Source: three-view drawing plus pictorial views. Frame: mm from the lowest corner of the part. Coordinates: 2 decimals unless noted, no trailing zeros. Write each loop counter-clockwise with the first axis right and the second up, starting at its lowest first coordinate (ties: lowest second). Pieces come first, ordered by that corner, then holes. Notation, with made-up numbers: (8, 69.25) -> (17, 69.25) arc R7 cw to (17, 80.25) -> close; hole circle Ø11 at (60.25, -6). An arc over 180 degrees is marked (long way). Write item = value, one per line.
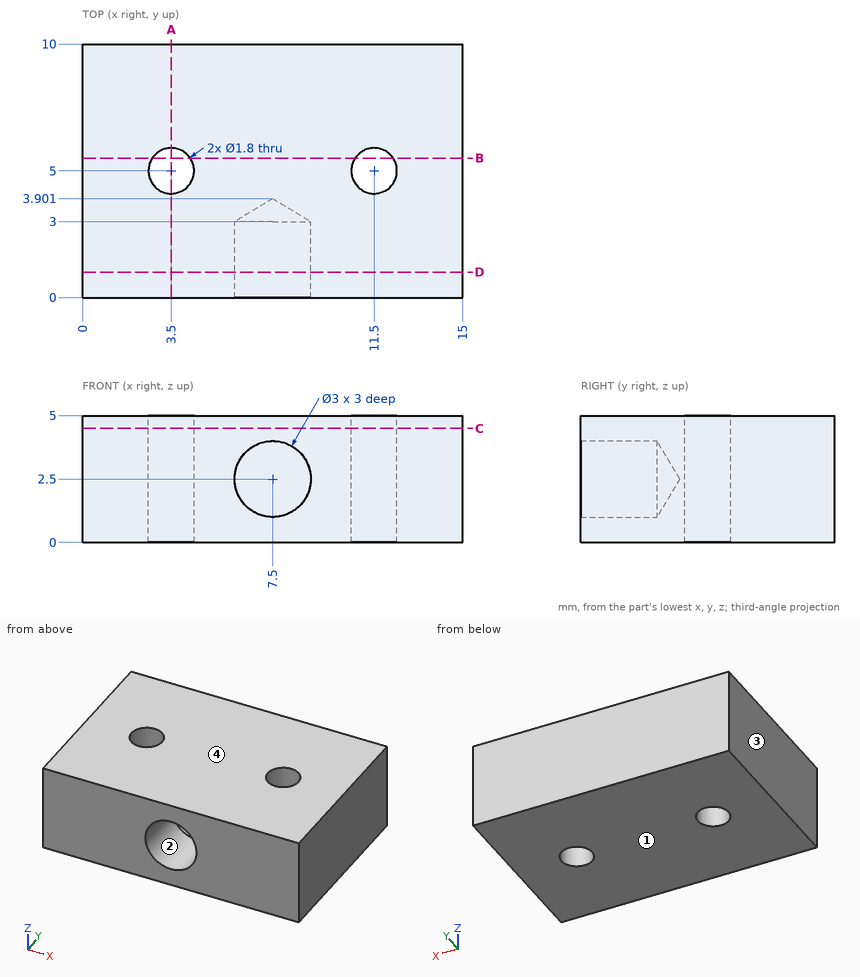
1) Cut plane A-A, the plane x = 3.5. Output: boundary loops of the cut face in (y, z), and give its area (3 significant figures).
Answer block:
outline = (0, 0) -> (4.1, 0) -> (4.1, 5) -> (0, 5) -> close; (5.9, 0) -> (10, 0) -> (10, 5) -> (5.9, 5) -> close
area = 41.0 mm2
2) Pull-direction query (Z, two-part tool) for the marked faces 1, 2, 3 and 4; classes: +Z half, -Z half, draft (parallel to the pull), parting line (faces both ways), or undercut.
Answer block:
face_1 = -Z half
face_2 = undercut
face_3 = draft
face_4 = +Z half
3) Material intervals for probe 1 along Y at (x, z) = (11.5, 2.15); probe 2 along Z at (x, y) = (7.5, 2.2); probe 3 along X at (y, z) = (2, 2.2), sorted ascending. Write a range as [from, to].
Answer block:
probe_1 = [0, 4.1], [5.9, 10]
probe_2 = [0, 1], [4, 5]
probe_3 = [0, 6.03], [8.97, 15]
4) Cut plane D-D, the plane y = 1. Output: boundary loops of the cut face in (x, z).
Answer block:
outline = (0, 0) -> (15, 0) -> (15, 5) -> (0, 5) -> close; hole circle Ø3 at (7.5, 2.5)
5) Cut plane C-C, the plane z = 4.5. Output: boundary loops of the cut face in (x, y), and give its area (3 significant figures).
Answer block:
outline = (0, 0) -> (15, 0) -> (15, 10) -> (0, 10) -> close; hole circle Ø1.8 at (3.5, 5); hole circle Ø1.8 at (11.5, 5)
area = 145 mm2
6) Cut plane B-B, the plane y = 5.5. Output: boundary loops of the cut face in (x, z).
Answer block:
outline = (0, 0) -> (2.75, 0) -> (2.75, 5) -> (0, 5) -> close; (4.25, 0) -> (10.75, 0) -> (10.75, 5) -> (4.25, 5) -> close; (12.25, 0) -> (15, 0) -> (15, 5) -> (12.25, 5) -> close
